```python
from build123d import *

# Parameters (mm, degrees)
SKETCH1_W           = 50.8
SKETCH1_H           = 25.4
SKETCH1_W_2         = 47.625
SKETCH1_H_2         = 22.225
BOSS_EXTRUDE1_DEPTH = 323.85
SKETCH2_R           = 14.305600685
CUT_EXTRUDE1_DEPTH  = 26.4
SKETCH4_R           = 12.637898421
CUT_EXTRUDE3_DEPTH  = 26.4


with BuildPart() as part:
    # Sketch1 → Boss-Extrude1 (new body)
    with BuildSketch(Plane.XY):
        with Locations((18.190104167, -7.24296875)):
            Rectangle(SKETCH1_W, SKETCH1_H)
        with Locations((18.190104167, -7.24296875)):
            Rectangle(SKETCH1_W_2, SKETCH1_H_2, mode=Mode.SUBTRACT)
    extrude(amount=BOSS_EXTRUDE1_DEPTH)

    # Sketch2 → Cut-Extrude1 (cut, through all)
    with BuildSketch(Plane(origin=(0, 5.45703125, 0), x_dir=(1, 0, 0), z_dir=(0, 1, 0))):
        with Locations((18.190104167, -25.4)):
            Circle(SKETCH2_R)
    extrude(amount=-CUT_EXTRUDE1_DEPTH, mode=Mode.SUBTRACT)

    # Sketch4 → Cut-Extrude3 (cut, through all)
    with BuildSketch(Plane(origin=(0, 5.45703125, 0), x_dir=(1, 0, 0), z_dir=(0, 1, 0))):
        with Locations((18.190104167, -218.186)):
            Circle(SKETCH4_R)
    extrude(amount=-CUT_EXTRUDE3_DEPTH, mode=Mode.SUBTRACT)


solid = part.part
```
Here's how the part is built. I have some questions about the finished solid (model axes, mm). A direction names the side the tool comes from. Give positions to 0.01 mm unless a question says otherwise; leave off trailing zeros. Loops run counter-clockwise (first coordinate to the right, second up) from the corner with the lowest first, then second, coordinate; pieces in that order, holes last. Notation, with made-up numbers: M 1.25,12 L 7.25,12 A22 ccw 7.25,21 Z; hole C 70.5,-4.5 d3. An arc over 180 degrees is marked long. Put each result on its own line as item: value. Start each with the question number.
(1) For faces 1 (the flat face through (43.59, -7, 160)), 2 (the flat face through (18, -18.355, 160)), which set-ups out of +Z, -Z, +X, -X, +Y, -Y let a thin tool reach every point of the face, with its end or its side?
(2) I want a section at B-B on x = 0.5. Please give me the cut outline in (y, z), then the cut area to 3 significant figures.
(3) I want a section at D-D on x = 18. Please give me the cut outline in (y, z), then the cut area to 3 significant figures.
(4) If we mould it in two halves opening along Z, with no side actions, what happens to faces 3 (the flat face through (18, -19, 0)), 4 (the flat face through (18, 5.457, 160)), 5 (the cylindrical face through (24.02, 4.67, 229.4))? For each: +Z half, -Z half, draft (parallel to the pull), parting line (faces both ways), or undercut.
(5) I want a section at A-A on z = 25.4. Please give me the cut outline in (x, y), then the cut area to 3 significant figures.
(6) I want a section at C-C on y = -9.5. Please give me the cut outline in (x, z), then the cut area to 3 significant figures.
(7) I need wall thicknesses on line 1 along Y through (x, z) = (10, 271); line 2 along X through (y, z) = (4.5, 25.4); line 3 along X through (y, z) = (-16.5, 56.5). Which ranges of each line are inside material? Lowest first, please. Write a range as [from, to].
Answer block:
1. face 1: +Z, -Z, +X, +Y, -Y
1. face 2: +Z, -Z
2. outline: M -19.94,0 L -18.36,0 L -18.36,323.85 L -19.94,323.85 Z; M 3.87,0 L 5.46,0 L 5.46,323.85 L 3.87,323.85 Z
2. area: 1,030 mm^2
3. outline: M -19.94,0 L -18.36,0 L -18.36,11.1 L -19.94,11.1 Z; M -19.94,39.7 L -18.36,39.7 L -18.36,205.55 L -19.94,205.55 Z; M -19.94,230.82 L -18.36,230.82 L -18.36,323.85 L -19.94,323.85 Z; M 3.87,0 L 5.46,0 L 5.46,11.1 L 3.87,11.1 Z; M 3.87,39.7 L 5.46,39.7 L 5.46,205.55 L 3.87,205.55 Z; M 3.87,230.82 L 5.46,230.82 L 5.46,323.85 L 3.87,323.85 Z
3. area: 857 mm^2
4. face 3: -Z half
4. face 4: draft
4. face 5: undercut
5. outline: M -7.21,-19.94 L 3.88,-19.94 L 3.88,-18.36 L -5.62,-18.36 L -5.62,3.87 L 3.88,3.87 L 3.88,5.46 L -7.21,5.46 Z; M 32.5,-19.94 L 43.59,-19.94 L 43.59,5.46 L 32.5,5.46 L 32.5,3.87 L 42,3.87 L 42,-18.36 L 32.5,-18.36 Z
5. area: 141 mm^2
6. outline: M -7.21,0 L -5.62,0 L -5.62,323.85 L -7.21,323.85 Z; M 42,0 L 43.59,0 L 43.59,323.85 L 42,323.85 Z
6. area: 1,030 mm^2
7. line 1: [-19.94, -18.36], [3.87, 5.46]
7. line 2: [-7.21, 3.88], [32.5, 43.59]
7. line 3: [-7.21, -5.62], [42, 43.59]
